from build123d import *

# Parameters (mm, degrees)
SKETCH_1_W          = 140
SKETCH_1_H          = 65
EXTRUDE_1_DEPTH     = 2
SKETCH_2_W          = 4
SKETCH_2_H          = 40
EXTRUDE_2_DEPTH     = 2
CUT_EXTRUDE_1_DEPTH = 2
SKETCH_4_R          = 1.6
CUT_EXTRUDE_2_DEPTH = 2
SKETCH_5_R          = 1.6
CUT_EXTRUDE_3_DEPTH = 2
CUT_EXTRUDE_4_DEPTH = 81.847077869
FILLET_1_R          = 3
EXTRUDE_3_DEPTH     = 2


with BuildPart() as part:
    # 草图1 → 凸台-拉伸1 (new body)
    with BuildSketch(Plane.XY):
        Rectangle(SKETCH_1_W, SKETCH_1_H)
    extrude(amount=EXTRUDE_1_DEPTH)

    # 草图2 → 凸台-拉伸2 (add)
    with BuildSketch(Plane.XY.offset(2)):
        with Locations((-72, 2.5)):
            Rectangle(SKETCH_2_W, SKETCH_2_H)
        with Locations((72, 2.5)):
            Rectangle(SKETCH_2_W, SKETCH_2_H)
    extrude(amount=-EXTRUDE_2_DEPTH)

    # 草图3 → 切除-拉伸1 (cut)
    with BuildSketch(Plane.XY.offset(2)):
        with BuildLine():
            Line((-65, -20), (-65, 20))
            ThreePointArc((-65, 20), (-60, 25), (-55, 20))
            Line((-55, 20), (-55, -20))
            ThreePointArc((-55, -20), (-60, -25), (-65, -20))
        make_face()
        with BuildLine():
            Line((-50, -20), (-50, 20))
            ThreePointArc((-50, 20), (-45, 25), (-40, 20))
            Line((-40, 20), (-40, -20))
            ThreePointArc((-40, -20), (-45, -25), (-50, -20))
        make_face()
        with BuildLine():
            Line((-35, -20), (-35, 20))
            ThreePointArc((-35, 20), (-30, 25), (-25, 20))
            Line((-25, 20), (-25, -20))
            ThreePointArc((-25, -20), (-30, -25), (-35, -20))
        make_face()
        with BuildLine():
            Line((-20, -20), (-20, 20))
            ThreePointArc((-20, 20), (-15, 25), (-10, 20))
            Line((-10, 20), (-10, -20))
            ThreePointArc((-10, -20), (-15, -25), (-20, -20))
        make_face()
        with BuildLine():
            Line((-5, -20), (-5, 20))
            ThreePointArc((-5, 20), (0, 25), (5, 20))
            Line((5, 20), (5, -20))
            ThreePointArc((5, -20), (0, -25), (-5, -20))
        make_face()
        with BuildLine():
            Line((10, -20), (10, 20))
            ThreePointArc((10, 20), (15, 25), (20, 20))
            Line((20, 20), (20, -20))
            ThreePointArc((20, -20), (15, -25), (10, -20))
        make_face()
        with BuildLine():
            Line((25, -20), (25, 20))
            ThreePointArc((25, 20), (30, 25), (35, 20))
            Line((35, 20), (35, -20))
            ThreePointArc((35, -20), (30, -25), (25, -20))
        make_face()
        with BuildLine():
            Line((40, -20), (40, 20))
            ThreePointArc((40, 20), (45, 25), (50, 20))
            Line((50, 20), (50, -20))
            ThreePointArc((50, -20), (45, -25), (40, -20))
        make_face()
        with BuildLine():
            Line((55, -20), (55, 20))
            ThreePointArc((55, 20), (60, 25), (65, 20))
            Line((65, 20), (65, -20))
            ThreePointArc((65, -20), (60, -25), (55, -20))
        make_face()
    extrude(amount=-CUT_EXTRUDE_1_DEPTH, mode=Mode.SUBTRACT)

    # 草图4 → 切除-拉伸2 (cut)
    with BuildSketch(Plane(origin=(0, 0, 0), x_dir=(-1, 0, 0), z_dir=(0, 0, -1))):
        with Locations((-40, -30)):
            Circle(SKETCH_4_R)
        with Locations(Location((40, -30, 0), (0, 0, 180))):
            Circle(SKETCH_4_R)
        with Locations((40, 30)):
            Circle(SKETCH_4_R)
        with Locations(Location((-40, 30, 0), (0, 0, 180))):
            Circle(SKETCH_4_R)
    extrude(amount=-CUT_EXTRUDE_2_DEPTH, mode=Mode.SUBTRACT)

    # 草图5 → 切除-拉伸3 (cut)
    with BuildSketch(Plane(origin=(0, 0, 0), x_dir=(-1, 0, 0), z_dir=(0, 0, -1))):
        with Locations((-65, -29)):
            Circle(SKETCH_5_R)
        with Locations(Location((-65, 29, 0), (0, 0, 180))):
            Circle(SKETCH_5_R)
        with Locations(Location((65, -29, 0), (0, 0, 180))):
            Circle(SKETCH_5_R)
        with Locations((65, 29)):
            Circle(SKETCH_5_R)
    extrude(amount=-CUT_EXTRUDE_3_DEPTH, mode=Mode.SUBTRACT)

    # 草图6 → 切除-拉伸4 (cut, through all)
    with BuildSketch(Plane(origin=(0, 0, 0), x_dir=(-1, 0, 0), z_dir=(0, 0, -1))):
        with BuildLine():
            Line((-6, -32.5), (6, -32.5))
            ThreePointArc((6, -32.5), (0, -26.5), (-6, -32.5))
        make_face()
    extrude(amount=-CUT_EXTRUDE_4_DEPTH, mode=Mode.SUBTRACT)

    # 圆角1
    fillet_1_edges = [part.edges().sort_by_distance(p)[0] for p in [
        (6, -32.5, 1),
        (-6, -32.5, 1),
    ]]
    fillet(fillet_1_edges, radius=FILLET_1_R)

    # 草图7 → 凸台-拉伸3 (add, through all)
    with BuildSketch(Plane(origin=(0, 0, 0), x_dir=(-1, 0, 0), z_dir=(0, 0, -1))):
        with BuildLine():
            Line((5, -15), (5, -20))
            ThreePointArc((5, -20), (0, -25), (-5, -20))
            Line((-5, -20), (-5, -15))
            ThreePointArc((-5, -15), (0, -20), (5, -15))
        make_face()
    extrude(amount=-EXTRUDE_3_DEPTH)


solid = part.part
Part model, mm, in its own coordinate system. Coordinates: 2 decimals unless noted, no trailing zeros. Loops run counter-clockwise (first coordinate to the right, second up) from the corner with the lowest first, then second, coordinate; pieces in that order, holes last. Notation, with made-up numbers: M 52.5,-2 L 70.5,-2 A31 ccw 70.5,36 Z; hole C -14,28 d3. An arc over 180 degrees is marked long. Use a Markdown table: item, result. Add a question column.
Q1. Cut at B-B (y = -6). Give the number of separate pieces and of enclosed holes in the cut face, and give its area (3 significant figures).
Q2. Mould opens along Y. For faces 1 (the flat face through (-50.4, 0.5, 0)), 2 (the cylindrical face through (40.208, -28.414, 0.986)), 3 (the cylindrical face through (-0.1, -26.5, 1)) say: +Y half, -Y half, draft (parallel to the pull), parting line (faces both ways), or undercut.
Q3. Probe L1, parallel to X at y = 27, z = 1.2; L2, parallel to Y at x = -33, z = 1.15; L3, parallel to Y at x = -3.5, z = 0.25. List the from-to ranges inside material, lowest first.
Q4. Pin check, flat tip, straight feed: P1, Ø1, axis at x = -71.5, z = 1, coming from the +Y side. Stop position of the tip, or through.
Q5. Cut at A-A (x = -15). Write the cut outline in (y, z), and give its area (3 significant figures).
Worked out:
| question | item | result |
|---|---|---|
| 1 | separate pieces | 10 |
| 1 | enclosed holes | 0 |
| 1 | area | 116 mm2 |
| 2 | face 1 | draft |
| 2 | face 2 | undercut |
| 2 | face 3 | -Y half |
| 3 | L1 | x = -70 to 70 |
| 3 | L2 | y = -32.5 to -24, 24 to 32.5 |
| 3 | L3 | y = -27.63 to -18.57, 23.57 to 32.5 |
| 4 | P1 | stops at y = 22.5 |
| 5 | outline | M -32.5,0 L -25,0 L -25,2 L -32.5,2 Z; M 25,0 L 32.5,0 L 32.5,2 L 25,2 Z |
| 5 | area | 30.0 mm2 |
